```python
from build123d import *

# Parameters (mm, degrees)
F0_W         = 25
F0_H         = 25
F1_DEPTH     = 12.5
F2_R         = 1.5
F3_DEPTH     = 25
F4_R         = 1.5
F5_DEPTH     = 25.001
F6_R         = 1.5
F7_DEPTH     = 25.001
F8_T1_DEPTH  = 32.5014485681
F8_T3_DEPTH  = 14.9980686292
F8_T5_DEPTH  = 14.9980686292
F8_S9_W      = 5.5015022539
F8_S9_H      = 5.5015022539
F8_T10_DEPTH = 5.501502254
F8_S15_W     = 5.5015022539
F8_S15_H     = 5.5015022539
F8_T16_DEPTH = 5.501502254
F8_S21_W     = 5.5015022539
F8_S21_H     = 5.5015022539
F8_T22_DEPTH = 5.501502254
F8_S27_W     = 5.5015022539
F8_S27_H     = 5.5015022539
F8_T28_DEPTH = 5.501502254
F10_R        = 1.5
F11_DEPTH    = 31.8208051534
F13_R        = 1.5
F14_DEPTH    = 31.8208052241


# Not quite as in the source:
# - a fillet or chamfer that OpenCascade refuses, or shapes differently, is made with other operations: its cross-section is extruded or revolved along the edge and cut away or added


with BuildPart() as f1:
    # F0 (on Front) → F1 (new body, symmetric)
    with BuildSketch(Plane.XZ):
        Rectangle(F0_W, F0_H)
    extrude(amount=F1_DEPTH, both=True)

    # F2 (on face) → F3 (cut, through all)
    with BuildSketch(Plane.XZ.offset(12.5)):
        Circle(F2_R)
    extrude(amount=-F3_DEPTH, mode=Mode.SUBTRACT)

    # F4 (on face) → F5 (cut, through all)
    with BuildSketch(Plane(origin=(0, 0, -12.5), x_dir=(1, 0, 0), z_dir=(0, 0, -1))):
        Circle(F4_R)
    extrude(amount=-F5_DEPTH, mode=Mode.SUBTRACT)

    # F6 (on face) → F7 (cut, through all)
    with BuildSketch(Plane(origin=(-12.5, 0, 0), x_dir=(0, -1, 0), z_dir=(-1, 0, 0))):
        Circle(F6_R)
    extrude(amount=-F7_DEPTH, mode=Mode.SUBTRACT)

    # F8: fillet of radius 5 on 8 edges, made by hand

    # F8_s2 → F8_t1 (cut)
    with BuildSketch(Plane.XY.offset(-25.0024142536)):
        with BuildLine():
            ThreePointArc((7.4990343146, -12.5004), (11.0355339059, -11.0355339059), (12.5004, -7.4990343146))
            Line((12.5004, -7.4990343146), (13.0005365685, -7.4990343146))
            ThreePointArc((13.0005365685, -7.4990343146), (13.0001365685, -9.9995171573), (13.0001365685, -12.5))
            Line((13.0001365685, -12.5), (12.5, -13.0001365685))
            ThreePointArc((12.5, -13.0001365685), (9.9995171573, -13.0001365685), (7.4990343146, -13.0005365685))
            Line((7.4990343146, -13.0005365685), (7.4990343146, -12.5004))
        make_face()
        with BuildLine():
            ThreePointArc((-12.5004, 7.4990343146), (-11.0355339059, 11.0355339059), (-7.4990343146, 12.5004))
            Line((-7.4990343146, 12.5004), (-7.4990343146, 13.0005365685))
            ThreePointArc((-7.4990343146, 13.0005365685), (-9.9995171573, 13.0001365685), (-12.5, 13.0001365685))
            Line((-12.5, 13.0001365685), (-13.0001365685, 12.5))
            ThreePointArc((-13.0001365685, 12.5), (-13.0001365685, 9.9995171573), (-13.0005365685, 7.4990343146))
            Line((-13.0005365685, 7.4990343146), (-12.5004, 7.4990343146))
        make_face()
        with BuildLine():
            ThreePointArc((-12.5004, -7.4990343146), (-11.0355339059, -11.0355339059), (-7.4990343146, -12.5004))
            Line((-7.4990343146, -12.5004), (-7.4990343146, -13.0005365685))
            ThreePointArc((-7.4990343146, -13.0005365685), (-9.9995171573, -13.0001365685), (-12.5, -13.0001365685))
            Line((-12.5, -13.0001365685), (-13.0001365685, -12.5))
            ThreePointArc((-13.0001365685, -12.5), (-13.0001365685, -9.9995171573), (-13.0005365685, -7.4990343146))
            Line((-13.0005365685, -7.4990343146), (-12.5004, -7.4990343146))
        make_face()
        with BuildLine():
            ThreePointArc((7.4990343146, 12.5004), (11.0355339059, 11.0355339059), (12.5004, 7.4990343146))
            Line((12.5004, 7.4990343146), (13.0005365685, 7.4990343146))
            ThreePointArc((13.0005365685, 7.4990343146), (13.0001365685, 9.9995171573), (13.0001365685, 12.5))
            Line((13.0001365685, 12.5), (12.5, 13.0001365685))
            ThreePointArc((12.5, 13.0001365685), (9.9995171573, 13.0001365685), (7.4990343146, 13.0005365685))
            Line((7.4990343146, 13.0005365685), (7.4990343146, 12.5004))
        make_face()
    extrude(amount=F8_T1_DEPTH, mode=Mode.SUBTRACT)

    # F8_s4 → F8_t3 (cut)
    with BuildSketch(Plane.XZ.offset(-7.4990343146)):
        with BuildLine():
            ThreePointArc((7.4990343146, 12.5004), (11.0355339059, 11.0355339059), (12.5004, 7.4990343146))
            Line((12.5004, 7.4990343146), (13.0005365685, 7.4990343146))
            ThreePointArc((13.0005365685, 7.4990343146), (13.0001365685, 9.9995171573), (13.0001365685, 12.5))
            Line((13.0001365685, 12.5), (12.5, 13.0001365685))
            ThreePointArc((12.5, 13.0001365685), (9.9995171573, 13.0001365685), (7.4990343146, 13.0005365685))
            Line((7.4990343146, 13.0005365685), (7.4990343146, 12.5004))
        make_face()
        with BuildLine():
            ThreePointArc((-12.5004, 7.4990343146), (-11.0355339059, 11.0355339059), (-7.4990343146, 12.5004))
            Line((-7.4990343146, 12.5004), (-7.4990343146, 13.0005365685))
            ThreePointArc((-7.4990343146, 13.0005365685), (-9.9995171573, 13.0001365685), (-12.5, 13.0001365685))
            Line((-12.5, 13.0001365685), (-13.0001365685, 12.5))
            ThreePointArc((-13.0001365685, 12.5), (-13.0001365685, 9.9995171573), (-13.0005365685, 7.4990343146))
            Line((-13.0005365685, 7.4990343146), (-12.5004, 7.4990343146))
        make_face()
    extrude(amount=F8_T3_DEPTH, mode=Mode.SUBTRACT)

    # F8_s6 → F8_t5 (cut)
    with BuildSketch(Plane.YZ.offset(-7.4990343146)):
        with BuildLine():
            ThreePointArc((12.5004, 7.4990343146), (11.0355339059, 11.0355339059), (7.4990343146, 12.5004))
            Line((7.4990343146, 12.5004), (7.4990343146, 13.0005365685))
            ThreePointArc((7.4990343146, 13.0005365685), (9.9995171573, 13.0001365685), (12.5, 13.0001365685))
            Line((12.5, 13.0001365685), (13.0001365685, 12.5))
            ThreePointArc((13.0001365685, 12.5), (13.0001365685, 9.9995171573), (13.0005365685, 7.4990343146))
            Line((13.0005365685, 7.4990343146), (12.5004, 7.4990343146))
        make_face()
        with BuildLine():
            ThreePointArc((-7.4990343146, 12.5004), (-11.0355339059, 11.0355339059), (-12.5004, 7.4990343146))
            Line((-12.5004, 7.4990343146), (-13.0005365685, 7.4990343146))
            ThreePointArc((-13.0005365685, 7.4990343146), (-13.0001365685, 9.9995171573), (-13.0001365685, 12.5))
            Line((-13.0001365685, 12.5), (-12.5, 13.0001365685))
            ThreePointArc((-12.5, 13.0001365685), (-9.9995171573, 13.0001365685), (-7.4990343146, 13.0005365685))
            Line((-7.4990343146, 13.0005365685), (-7.4990343146, 12.5004))
        make_face()
    extrude(amount=F8_T5_DEPTH, mode=Mode.SUBTRACT)


with BuildPart() as f8_tool8:
    # F8_s9 → F8_t10 (new body)
    with BuildSketch(Plane.XY.offset(7.4990343146)):
        with Locations((10.2497854415, -10.2497854415)):
            Rectangle(F8_S9_W, F8_S9_H)
    extrude(amount=F8_T10_DEPTH)

    # F8_s11 → F8_t12 (revolve, cut)
    with BuildSketch(Plane(origin=(7.4990343146, -7.4990343146, 7.4990343146), x_dir=(-0.7071067812, 0.7071067812, 0), z_dir=(0.7071067812, 0.7071067812, 0))):
        with BuildLine():
            ThreePointArc((0, -5.0013656854), (5.0013656854, 0), (0, 5.0013656854))
            Line((0, 5.0013656854), (0, -5.0013656854))
        make_face()
    revolve(axis=Axis((7.4990343146, -7.4990343146, 7.4990343146), (0, 0, 1)), mode=Mode.SUBTRACT)


with BuildPart() as f1_1:
    add(f1.part)

    # F8_t7: cut F8_tool8
    add(f8_tool8.part, mode=Mode.SUBTRACT)


with BuildPart() as f8_tool14:
    # F8_s15 → F8_t16 (new body)
    with BuildSketch(Plane.XZ.offset(-7.4990343146)):
        with Locations((10.2497854415, 10.2497854415)):
            Rectangle(F8_S15_W, F8_S15_H)
    extrude(amount=-F8_T16_DEPTH)

    # F8_s17 → F8_t18 (revolve, cut)
    with BuildSketch(Plane(origin=(7.4990343146, 7.4990343146, 7.4990343146), x_dir=(-0.7071067812, 0, -0.7071067812), z_dir=(0.7071067812, 0, -0.7071067812))):
        with BuildLine():
            ThreePointArc((0, -5.0013656854), (5.0013656854, 0), (0, 5.0013656854))
            Line((0, 5.0013656854), (0, -5.0013656854))
        make_face()
    revolve(axis=Axis((7.4990343146, 7.4990343146, 7.4990343146), (0, 1, 0)), mode=Mode.SUBTRACT)


with BuildPart() as f1_2:
    add(f1_1.part)

    # F8_t13: cut F8_tool14
    add(f8_tool14.part, mode=Mode.SUBTRACT)


with BuildPart() as f8_tool20:
    # F8_s21 → F8_t22 (new body)
    with BuildSketch(Plane.YZ.offset(-7.4990343146)):
        with Locations((10.2497854415, 10.2497854415)):
            Rectangle(F8_S21_W, F8_S21_H)
    extrude(amount=-F8_T22_DEPTH)

    # F8_s23 → F8_t24 (revolve, cut)
    with BuildSketch(Plane(origin=(-7.4990343146, 7.4990343146, 7.4990343146), x_dir=(0, -0.7071067812, -0.7071067812), z_dir=(0, 0.7071067812, -0.7071067812))):
        with BuildLine():
            ThreePointArc((0, -5.0013656854), (5.0013656854, 0), (0, 5.0013656854))
            Line((0, 5.0013656854), (0, -5.0013656854))
        make_face()
    revolve(axis=Axis((-7.4990343146, 7.4990343146, 7.4990343146), (-1, 0, 0)), mode=Mode.SUBTRACT)


with BuildPart() as f1_3:
    add(f1_2.part)

    # F8_t19: cut F8_tool20
    add(f8_tool20.part, mode=Mode.SUBTRACT)


with BuildPart() as f8_tool26:
    # F8_s27 → F8_t28 (new body)
    with BuildSketch(Plane.YZ.offset(-7.4990343146)):
        with Locations((-10.2497854415, 10.2497854415)):
            Rectangle(F8_S27_W, F8_S27_H)
    extrude(amount=-F8_T28_DEPTH)

    # F8_s29 → F8_t30 (revolve, cut)
    with BuildSketch(Plane(origin=(-7.4990343146, -7.4990343146, 7.4990343146), x_dir=(0, 0.7071067812, -0.7071067812), z_dir=(0, 0.7071067812, 0.7071067812))):
        with BuildLine():
            ThreePointArc((0, -5.0013656854), (5.0013656854, 0), (0, 5.0013656854))
            Line((0, 5.0013656854), (0, -5.0013656854))
        make_face()
    revolve(axis=Axis((-7.4990343146, -7.4990343146, 7.4990343146), (-1, 0, 0)), mode=Mode.SUBTRACT)


with BuildPart() as f1_4:
    add(f1_3.part)

    # F8_t25: cut F8_tool26
    add(f8_tool26.part, mode=Mode.SUBTRACT)

    # F10 (on face) → F11 (cut, through all)
    with BuildSketch(Plane(origin=(10, 10, 0), x_dir=(-0.7071067812, 0.7071067812, 0), z_dir=(0.7071067812, 0.7071067812, 0))):
        Circle(F10_R)
    extrude(amount=-F11_DEPTH, mode=Mode.SUBTRACT)

    # F13 (on face) → F14 (cut, through all)
    with BuildSketch(Plane(origin=(10, -10, 0), x_dir=(0.7071067812, 0.7071067812, 0), z_dir=(0.7071067812, -0.7071067812, 0))):
        Circle(F13_R)
    extrude(amount=-F14_DEPTH, mode=Mode.SUBTRACT)


solid = f1_4.part
```
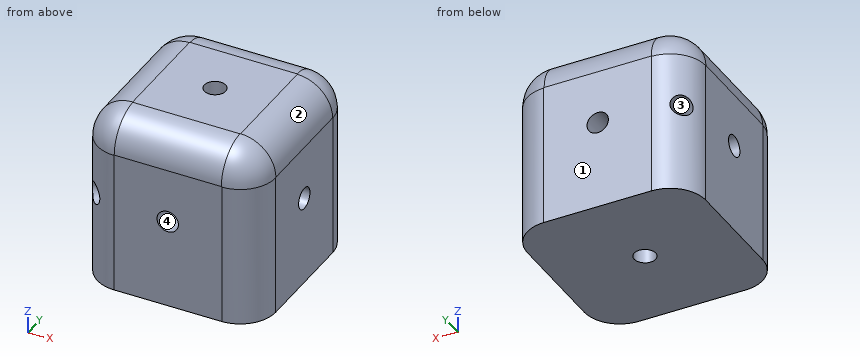
Input: part model. Units: mm. Frame: model coordinates. Face numbers are marked on the shaded views. Round coordinates to 2 decimals unless told otherwise and drop trailing zeros. Loops run counter-clockwise (first coordinate to the right, second up) from the corner with the lowest first, then second, coordinate; pieces in that order, holes last. Notation, with made-up numbers: (-37, 64.25) - (20, 64.25) arc R10 cw to (20, 78.25) - close; hole circle Ø3 at (-21.75, 66). An arc over 180 degrees is marked (long way). One line per item, written item: value. Start each with the question number.
(1) Contact query for flat-ended pins moving along their axis: P1, Ø1.8, axis at x = 0, y = 0, coming from the +Z side; P2, Ø4, axis at x = 0, z = 0, coming from the +Y side; P3, Ø1, axis at y = -8.5, z = 3.5, coming from the -X side. Output: stop coordinate, or through.
(2) Section B-B, the plane z = -5.75. Return loops of the section in (x, y).
(3) Draft query along Z for the marked faces 1, 2, 3 and 4. Return one class per face: +Z half, -Z half, draft (parallel to the pull), parting line (faces both ways), or undercut.
(4) Section A-A, the plane y = 0. Return loops of the section in (x, z), plus the area to 3 significant figures.
(5) Ray query, line 1 (Z direction, x = 0, y = -4.5); line 2 (X direction, y = 7.75, z = 0); line 3 (X direction, y = 7.5, z = 0). Return the intervals inside material, ascending. Write a range as [from, to].
(6) Section D-D, the plane z = 0.5. Count the separate pieces of the cut face and the enclosed holes in it, plus the area to 3 significant figures.
Results below:
1. P1: through
1. P2: y = 12.5
1. P3: x = -12.48
2. outline: (-12.5, -7.56) arc R5 ccw to (-7.56, -12.5) - (7.56, -12.5) arc R5 ccw to (12.5, -7.56) - (12.5, 7.56) arc R5 ccw to (7.56, 12.5) - (-7.56, 12.5) arc R5 ccw to (-12.5, 7.56) - close; hole circle Ø3 at (0, 0)
3. face 1: draft
3. face 2: +Z half
3. face 3: undercut
3. face 4: undercut
4. outline: (-12.5, -12.5) - (-1.5, -12.5) - (-1.5, -1.5) - (-12.5, -1.5) - close; (-12.5, 1.5) - (-1.5, 1.5) - (-1.5, 12.5) - (-7.56, 12.5) arc R5 ccw to (-12.5, 7.56) - close; (1.5, -12.5) - (12.5, -12.5) - (12.5, -1.5) - (1.5, -1.5) - close; (1.5, 1.5) - (12.5, 1.5) - (12.5, 7.56) arc R5 ccw to (7.56, 12.5) - (1.5, 12.5) - close
4. area: 473 mm^2
5. line 1: [-12.5, -1.5], [1.5, 12.5]
5. line 2: [-12.49, -9.87], [-5.63, -1.5], [1.5, 5.63], [9.87, 12.49]
5. line 3: [-12.5, -9.62], [-5.38, -1.5], [1.5, 5.38], [9.62, 12.5]
6. separate pieces: 6
6. enclosed holes: 0
6. area: 333 mm^2
